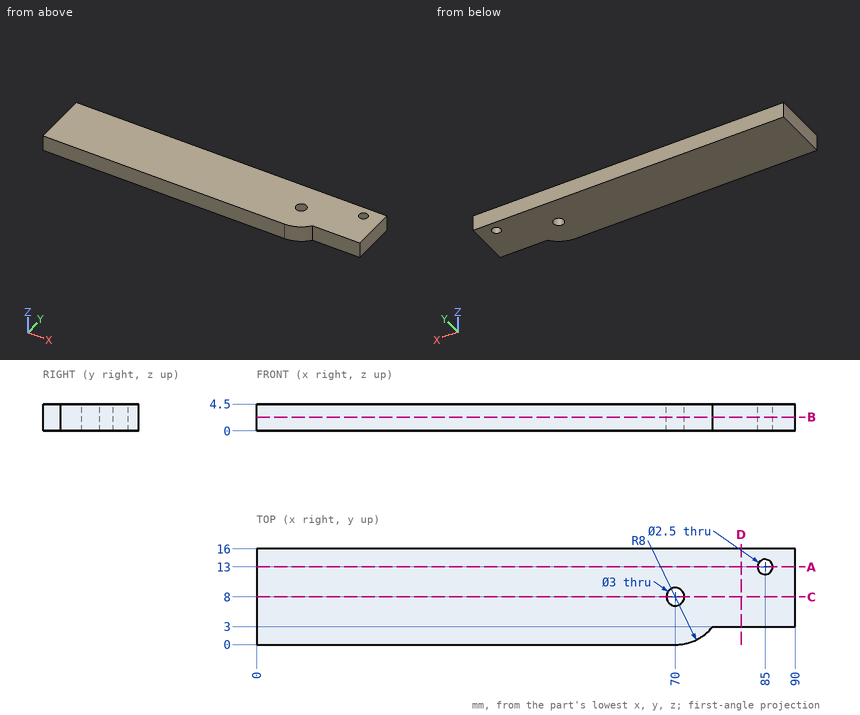
Design review of the part shown in the three views and the two pictorial views. Dimensions are in mm from the part's minimum x, y and z. Give positions to 0.01 mm unless a question says otherwise; leave off trailing zeros. Loops run counter-clockwise (first coordinate to the right, second up) from the corner with the lowest first, then second, coordinate; pieces in that order, holes last. Notation, with made-up numbers: (21, 20.25) -> (51, 20.25) arc R20 cw to (51, 41.25) -> close; hole circle Ø10 at (-32, -19). An arc over 180 degrees is marked (long way). Answer as a JSON object with one key per item and string values. Group by question number.
Q1. Take a section at B-B (z = 2.3). Write out the cut boundary in (x, y) (3 decimals), plus the area to 3 significant figures.
Q2. Take a section at A-A (y = 13). Write out the cut boundary in (x, z), plus the area to 3 significant figures.
Q3. Take a section at D-D (x = 81). Write out the cut boundary in (y, z).
Q4. Insertion check: pin 1 (2 mm diameter, centred on x = 80.5, z = 1.5, fed in from -Y). The pin has a flat end and moves straight along its axis. Give the tip position at first contact, or say it passes through.
Q5. Wall thickness on line 1 along X through (y, z) = (8, 3.4); line 2 along Y through (x, z) = (85, 2.55); line 3 along Y through (x, z) = (70, 2.1): over which ranges is each line inside the solid? List them lowest first.
Q6. Take a section at C-C (y = 8). Write out the cut boundary in (x, z).
Answer below:
{
 "1": {"outline": "(0, 0) -> (70, 0) arc R8 ccw to (76.245, 3) -> (90, 3) -> (90, 16) -> (0, 16) -> close; hole circle Ø3 at (70, 8); hole circle Ø2.5 at (85, 13)", "area": "1,380 mm2"},
 "2": {"outline": "(0, 0) -> (83.75, 0) -> (83.75, 4.5) -> (0, 4.5) -> close; (86.25, 0) -> (90, 0) -> (90, 4.5) -> (86.25, 4.5) -> close", "area": "394 mm2"},
 "3": {"outline": "(3, 0) -> (16, 0) -> (16, 4.5) -> (3, 4.5) -> close"},
 "4": {"pin 1": "stops at y = 3"},
 "5": {"line 1": "x = 0 to 68.5, 71.5 to 90", "line 2": "y = 3 to 11.75, 14.25 to 16", "line 3": "y = 0 to 6.5, 9.5 to 16"},
 "6": {"outline": "(0, 0) -> (68.5, 0) -> (68.5, 4.5) -> (0, 4.5) -> close; (71.5, 0) -> (90, 0) -> (90, 4.5) -> (71.5, 4.5) -> close"}
}
